Check sheet for the modelled part. Datum: model origin and axes. Units: mm. Give positions to 0.01 mm unless a question says otherwise; leave off trailing zeros. Loops run counter-clockwise (first coordinate to the right, second up) from the corner with the lowest first, then second, coordinate; pieces in that order, holes last. Notation, with made-up numbers: (-17.75, 36) - (24.25, 36) arc R16 ccw to (24.25, 41) - close; hole circle Ø1 at (60, 48.5). An arc over 180 degrees is marked (long way). Answer in a Markdown table with one row per item. Add a question column.
(1) Sectioned sample at B-B on x = 171. Enter the section's corners in (y, z).
(2) Sectioned sample at C-C on y = -3. State how many separate pieces and enclosed holes the cut face has, then the cut area to 3 significant figures.
(3) Sectioned sample at A-A on z = 41. Enter the section's corners in (x, y), then the cut area to 3 significant figures.
(4) Go/stop test with flat-tipped pins: P1, Ø1.5, axis at x = -149.5, y = -3.5, coming from the -Z side; P2, Ø5, axis at x = 126, y = -1.5, coming from the +Z side; P3, Ø1, axis at x = 129.5, z = -1.5, coming from the +Y side; P4, Ø2, axis at x = 129.5, y = -10, coming from the +Z side. Record where each tip stops, or that it passes through.
(5) Thickness scan on L1, parallel to Z at x = -137, y = -5; L2, parallel to Z at x = 8.5, y = -10.25; L3, parallel to X at y = -8, z = 25. Record the ranges inside material, lowest first.
(6) Sectioned sample at D-D on x = -120. Enter the section's corners in (y, z), then the cut area to 3 significant figures.
from build123d import *

# Parameters (mm, degrees)
F0_R     = 3.05
F1_DEPTH = 12.7


with BuildPart() as f1:
    # F0 (on Front) → F1 (new body)
    with BuildSketch(Plane.XZ):
        with BuildLine():
            ThreePointArc((51.488186, 26.23139), (30.193835, 49.269174), (0, 57.785112))
            ThreePointArc((0, 57.785112), (-30.193835, 49.269174), (-51.488186, 26.23139))
            Line((-51.488186, 26.23139), (-199.782062, 61.369492))
            Line((-199.782062, 61.369492), (-191.015825, 45.002539))
            Line((-191.015825, 45.002539), (-203.858078, 34.884386))
            Line((-203.858078, 34.884386), (-189.841708, 17.094403))
            Line((-189.841708, 17.094403), (-199.782062, 9.262597))
            Line((-199.782062, 9.262597), (-191.015825, -10.25812))
            Line((-191.015825, -10.25812), (-199.782062, -21.932906))
            Line((-199.782062, -21.932906), (-191.015825, -35.16433))
            Line((-191.015825, -35.16433), (-199.782062, -48.784915))
            Line((-199.782062, -48.784915), (-191.015825, -58.903065))
            Line((-191.015825, -58.903065), (-195.808372, -71.409119))
            Line((-195.808372, -71.409119), (-48.938758, -30.726488))
            ThreePointArc((-48.938758, -30.726488), (-27.960558, -50.570014), (0, -57.785112))
            ThreePointArc((0, -57.785112), (27.960558, -50.570014), (48.938758, -30.726488))
            Line((48.938758, -30.726488), (195.808372, -71.409119))
            Line((195.808372, -71.409119), (191.015825, -58.903065))
            Line((191.015825, -58.903065), (199.782062, -48.784915))
            Line((199.782062, -48.784915), (191.015825, -35.16433))
            Line((191.015825, -35.16433), (199.782062, -21.932906))
            Line((199.782062, -21.932906), (191.015825, -10.25812))
            Line((191.015825, -10.25812), (199.782062, 9.262597))
            Line((199.782062, 9.262597), (189.841708, 17.094403))
            Line((189.841708, 17.094403), (203.858078, 34.884386))
            Line((203.858078, 34.884386), (191.015825, 45.002539))
            Line((191.015825, 45.002539), (199.782062, 61.369492))
            Line((199.782062, 61.369492), (51.488186, 26.23139))
        make_face()
        with Locations((-178.394541, -10.163349)):
            Circle(F0_R, mode=Mode.SUBTRACT)
        with Locations((-136.394541, -10.163349)):
            Circle(F0_R, mode=Mode.SUBTRACT)
        with Locations((-87.394541, -10.163349)):
            Circle(F0_R, mode=Mode.SUBTRACT)
        with Locations((-38.394541, -10.163349)):
            Circle(F0_R, mode=Mode.SUBTRACT)
        with Locations((10.605459, -10.163349)):
            Circle(F0_R, mode=Mode.SUBTRACT)
        with Locations((73.605459, -10.163349)):
            Circle(F0_R, mode=Mode.SUBTRACT)
        with Locations((129.394541, -10.163349)):
            Circle(F0_R, mode=Mode.SUBTRACT)
        with Locations((-178.413816, 3.836376)):
            Circle(F0_R, mode=Mode.SUBTRACT)
        with Locations((-136.413816, 3.836376)):
            Circle(F0_R, mode=Mode.SUBTRACT)
        with Locations((-87.413816, 3.836376)):
            Circle(F0_R, mode=Mode.SUBTRACT)
        with Locations((-38.413816, 3.836376)):
            Circle(F0_R, mode=Mode.SUBTRACT)
        with Locations((10.586184, 3.836376)):
            Circle(F0_R, mode=Mode.SUBTRACT)
        with Locations((73.586184, 3.836376)):
            Circle(F0_R, mode=Mode.SUBTRACT)
        with Locations((129.375266, 3.836376)):
            Circle(F0_R, mode=Mode.SUBTRACT)
    extrude(amount=F1_DEPTH)


solid = f1.part
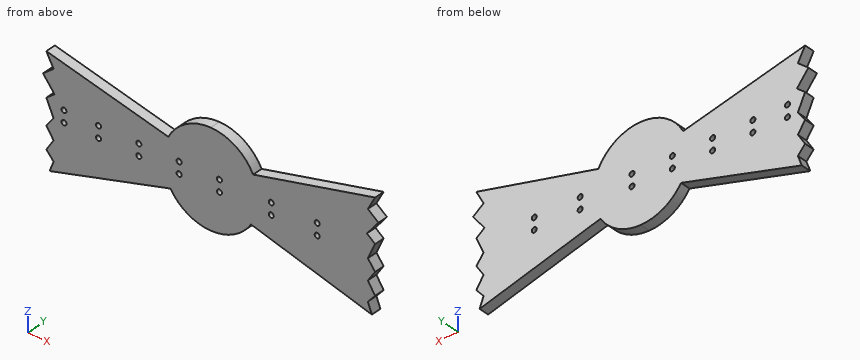
Reply:
| question | item | result |
|---|---|---|
| 1 | outline | (-12.7, -64.54) - (0, -64.54) - (0, 54.55) - (-12.7, 54.55) - close |
| 2 | separate pieces | 1 |
| 2 | enclosed holes | 14 |
| 2 | area | 36,900 mm^2 |
| 3 | outline | (-196.1, -12.7) - (-113.82, -12.7) - (-113.82, 0) - (-196.1, 0) - close; (-40.72, -12.7) - (40.72, -12.7) - (40.72, 0) - (-40.72, 0) - close; (113.82, -12.7) - (196.1, -12.7) - (196.1, 0) - (113.82, 0) - close |
| 3 | area | 3,120 mm^2 |
| 4 | P1 | z = -58.79 |
| 4 | P2 | z = 44.48 |
| 4 | P3 | y = 0 |
| 4 | P4 | z = 44.95 |
| 5 | L1 | -55.12 to -13.15, -7.17 to 0.84, 6.83 to 46.49 |
| 5 | L2 | -57.16 to -12.37, -7.96 to 1.61, 6.06 to 57.16 |
| 5 | L3 | -196.07 to 196.07 |
| 6 | outline | (-12.7, -50.41) - (0, -50.41) - (0, 42.47) - (-12.7, 42.47) - close |
| 6 | area | 1,180 mm^2 |
